```python
from build123d import *

# Parameters (mm, degrees)
F0_W     = 53
F0_H     = 123
F1_DEPTH = 7
F2_R     = 6
F3_SIZE  = 0.5
F4_T     = -2.5


with BuildPart() as f1:
    # F0 (on Top) → F1 (new body)
    with BuildSketch(Plane.XY):
        Rectangle(F0_W, F0_H)
    extrude(amount=F1_DEPTH)

    # F2
    f2_edges = [f1.edges().sort_by_distance(p)[0] for p in [
        (26.5, 61.5, 3.5),
        (-26.5, 61.5, 3.5),
        (26.5, -61.5, 3.5),
        (-26.5, -61.5, 3.5),
    ]]
    fillet(f2_edges, radius=F2_R)

    # F3
    f3_edges = [f1.edges().sort_by_distance(p)[0] for p in [
        (-26.5, 0, 7),
        (-24.742641, -59.742641, 7),
        (0, -61.5, 7),
        (24.742641, -59.742641, 7),
        (26.5, 0, 7),
        (24.742641, 59.742641, 7),
        (0, 61.5, 7),
        (-24.742641, 59.742641, 7),
    ]]
    chamfer(f3_edges, length=F3_SIZE)

    # F4
    f4_openings = [f1.faces().sort_by_distance(p)[0] for p in [
        (0, 0, 7),
    ]]
    offset(amount=F4_T, openings=f4_openings)


solid = f1.part
```
Work out the finished part from the listing and answer in its coordinate system (mm). A direction names the side the tool comes from. Coordinates: 2 decimals unless noted, no trailing zeros. Order: outer loops, then holes, each group sorted by start corner. A loop starts at its lowest first (then second) coordinate and runs counter-clockwise, first axis right, second up. Notation, with made-up numbers: (-17.5, -11.5) - (-2.5, -11.5) arc R21 ccw to (-2.5, 6.5) - close; hole circle Ø1 at (87.5, 77.25). An arc over 180 degrees is marked (long way). Answer as a JSON object with one key per item and string values.
1. A tool of negligible diameter and unlimited length cuts with its end or side. For faces 5 (the face through (-22.323, 57.284, 6.414)), 6 (the face through (0, -61.5, 3)), from which of +Z, -Z, +X, -X, +Y, -Y can it reach the whole face along a straight path? Write none if from no direction.
Output values:
{"face 5": "none", "face 6": "+Z, -Z, +X, -X, -Y"}
2. Find section A-A on x = -3.5. Determine the outline of the cut face in (y, z).
Output values:
{"outline": "(-61.5, 0) - (61.5, 0) - (61.5, 6.5) - (61, 7) - (57.46, 7) - (59, 5.46) - (59, 2.5) - (-59, 2.5) - (-59, 5.46) - (-57.46, 7) - (-61, 7) - (-61.5, 6.5) - close"}
3. Find section B-B on y = -42.5. Determine the outline of the cut face in (x, z).
Output values:
{"outline": "(-26.5, 0) - (26.5, 0) - (26.5, 6.5) - (26, 7) - (22.46, 7) - (24, 5.46) - (24, 2.5) - (-24, 2.5) - (-24, 5.46) - (-22.46, 7) - (-26, 7) - (-26.5, 6.5) - close"}
4. The mould has two halves that part along Z. Classify faces 1 (the face through (-24.789, -59.696, 3.296)), 2 (the face through (24.528, -59.441, 6.865)), 3 (the face through (-23, -57.95, 4)), 4 (the face through (22.95, -58, 4)): +Z half, -Z half, draft (parallel to the pull), parting line (faces both ways), or undercut.
Output values:
{"face 1": "draft", "face 2": "+Z half", "face 3": "undercut", "face 4": "undercut"}
5. This flat-tipped pin is pushed along its axis until it touches: P1, Ø24, axis at x = 5.5, y = 0, coming from the +Z side. Where does it stop, or does it pass through?
Output values:
{"P1": "stops at z = 2.5"}
6. Find section C-C on z = 4. Determine the outline of the cut face in (x, y).
Output values:
{"outline": "(-26.5, -55.5) arc R6 ccw to (-20.5, -61.5) - (20.5, -61.5) arc R6 ccw to (26.5, -55.5) - (26.5, 55.5) arc R6 ccw to (20.5, 61.5) - (-20.5, 61.5) arc R6 ccw to (-26.5, 55.5) - close; hole (-24, -55.5) arc R3.5 ccw to (-20.5, -59) - (20.5, -59) arc R3.5 ccw to (24, -55.5) - (24, 55.5) arc R3.5 ccw to (20.5, 59) - (-20.5, 59) arc R3.5 ccw to (-24, 55.5) - close"}
7. Consider line 1 (Y direction, x = -15, z = 5); line 2 (Z direction, x = 0.5, y = -12); line 3 (X direction, y = 49.5, z = 3.5). Determine where each line is inside the solid, lowest interval first.
Output values:
{"line 1": "y = -61.5 to -59, 59 to 61.5", "line 2": "z = 0 to 2.5", "line 3": "x = -26.5 to -24, 24 to 26.5"}
